from build123d import *

# Parameters (mm, degrees)
SKETCH1_W           = 320
SKETCH1_H           = 40
SKETCH1_R           = 10
BOSS_EXTRUDE1_DEPTH = 6
CUT_EXTRUDE2_DEPTH  = 10
CUT_EXTRUDE3_DEPTH  = 7


with BuildPart() as part:
    # Sketch1 → Boss-Extrude1 (new body)
    with BuildSketch(Plane(origin=(0, 0, 0), x_dir=(0, 0, -1), z_dir=(1, 0, 0))):
        Rectangle(SKETCH1_W, SKETCH1_H)
        with Locations((-140, 0)):
            Circle(SKETCH1_R, mode=Mode.SUBTRACT)
    extrude(amount=BOSS_EXTRUDE1_DEPTH)

    # Sketch2 → Cut-Extrude2 (cut)
    with BuildSketch(Plane.ZY):
        Polygon((54.001630689, -10), (72.183448871, 10), (90.365267053, -10), align=None)
        Polygon((22.305204555, 10), (58.668840919, 10), (40.487022737, -10), align=None)
        Polygon((-9.391221579, -10), (8.790596603, 10), (26.972414785, -10), align=None)
        Polygon((-4.724011349, 10), (-22.905829531, -10), (-41.087647713, 10), align=None)
        Polygon((-36.420437483, -10), (-72.784073847, -10), (-54.602255665, 10), align=None)
        Polygon((-68.116863617, 10), (-86.298681799, -10), (-104.48049998, 10), align=None)
        Polygon((-99.813289751, -10), (-136.176926114, -10), (-117.995107933, 10), align=None)
        Polygon((85.698056823, 10), (122.061693187, 10), (103.879875005, -10), align=None)
    extrude(amount=-CUT_EXTRUDE2_DEPTH, mode=Mode.SUBTRACT)

    # Sketch3 → Cut-Extrude3 (cut, through all)
    with BuildSketch(Plane.ZY):
        with BuildLine():
            Line((-146.04862835, 2.783997553), (-150.521776952, -2.136465909))
            Line((-150.521776952, -2.136465909), (-154.961417393, 1.899570855))
            Line((-154.961417393, 1.899570855), (-150.488268791, 6.820034317))
            ThreePointArc((-150.488268791, 6.820034317), (-149.34196576, 10.310877963), (-145.975842509, 11.783703228))
            Line((-145.975842509, 11.783703228), (-141.502693907, 16.70416669))
            Line((-141.502693907, 16.70416669), (-137.063053466, 12.668129926))
            Line((-137.063053466, 12.668129926), (-141.536202068, 7.747666464))
            ThreePointArc((-141.536202068, 7.747666464), (-142.682505099, 4.256822817), (-146.04862835, 2.783997553))
        make_face()
    extrude(amount=-CUT_EXTRUDE3_DEPTH, mode=Mode.SUBTRACT)


solid = part.part
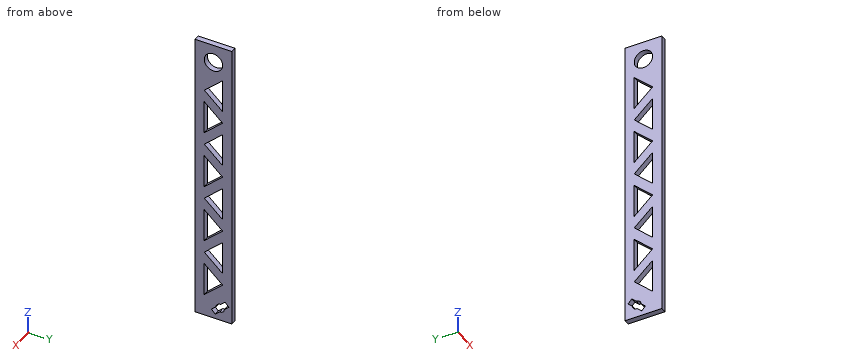
Work out the finished part from the listing and answer in its coordinate system (mm). Give positions to 0.01 mm unless a question says otherwise; leave off trailing zeros. Loops run counter-clockwise (first coordinate to the right, second up) from the corner with the lowest first, then second, coordinate; pieces in that order, holes last. Notation, with made-up numbers: (-38.5, 54.25) - (-3.5, 54.25) arc R20 ccw to (-3.5, 63.25) - close; hole circle Ø8 at (-17.5, 6). An arc over 180 degrees is marked (long way). Answer in a Markdown table with one row per item. Add a question column.
Q1. Consider line 1 along Y through (x, z) = (1.55, 140); line 2 along Y through (x, z) = (4.5, 26); line 3 along Z through (x, y) = (2.25, 16). Determine where each line is inside the solid, lowest interval first.
Q2. The part is cut by section D-D (z = -122). Determine the outline of the cut face in (x, y), and give its area (3 significant figures).
Q3. The part is cut by section B-B (x = 1.5). State how many separate pieces and enclosed holes the cut face has, and give its area (3 significant figures).
Q4. The part is cut by section A-A (z = 140). Determine the outline of the cut face in (x, y), and give its area (3 significant figures).
Solution:
| question | item | result |
|---|---|---|
| 1 | line 1 | y = -20 to -10, 10 to 20 |
| 1 | line 2 | y = -20 to -10, -8.93 to 5.94, 10 to 20 |
| 1 | line 3 | z = -160 to -142.14, -140.73 to 160 |
| 2 | outline | (0, -20) - (6, -20) - (6, -10) - (0, -10) - close; (0, 5.59) - (6, 5.59) - (6, 20) - (0, 20) - close |
| 2 | area | 146 mm² |
| 3 | separate pieces | 1 |
| 3 | enclosed holes | 10 |
| 3 | area | 9,440 mm² |
| 4 | outline | (0, -20) - (6, -20) - (6, -10) - (0, -10) - close; (0, 10) - (6, 10) - (6, 20) - (0, 20) - close |
| 4 | area | 120 mm² |
